from build123d import *

# Parameters (mm, degrees)
SKETCH1_R           = 13.75
SKETCH1_R_2         = 4.15
BOSS_EXTRUDE1_DEPTH = 2.5
SKETCH2_R           = 6.5
SKETCH2_R_2         = 4.15
BOSS_EXTRUDE2_DEPTH = 2.5
CUT_EXTRUDE1_DEPTH  = 21.077973005
FILLET1_R           = 0.5


with BuildPart() as part:
    # Sketch1 → Boss-Extrude1 (new body)
    with BuildSketch(Plane.XY):
        Circle(SKETCH1_R)
        Circle(SKETCH1_R_2, mode=Mode.SUBTRACT)
    extrude(amount=BOSS_EXTRUDE1_DEPTH)

    # Sketch2 → Boss-Extrude2 (add)
    with BuildSketch(Plane.XY.offset(2.5)):
        Circle(SKETCH2_R)
        Circle(SKETCH2_R_2, mode=Mode.SUBTRACT)
    extrude(amount=BOSS_EXTRUDE2_DEPTH)

    # Sketch5 → Cut-Extrude1 (cut, through all)
    with BuildSketch(Plane.XY):
        with BuildLine():
            Line((0, 12.75), (0, 7.5))
            ThreePointArc((0, 7.5), (5.303300859, 5.303300859), (7.5, 0))
            ThreePointArc((7.5, 0), (5.303300859, -5.303300859), (0, -7.5))
            Line((0, -7.5), (0, -12.75))
            ThreePointArc((0, -12.75), (9.01561146, -9.01561146), (12.75, 0))
            ThreePointArc((12.75, 0), (9.01561146, 9.01561146), (0, 12.75))
        make_face()
    extrude(amount=CUT_EXTRUDE1_DEPTH, mode=Mode.SUBTRACT)

    # Fillet1
    fillet1_edges = [part.edges().sort_by_distance(p)[0] for p in [
        (0, 7.5, 1.25),
        (0, -7.5, 1.25),
        (0, -12.75, 1.25),
        (0, 12.75, 1.25),
    ]]
    fillet(fillet1_edges, radius=FILLET1_R)


solid = part.part
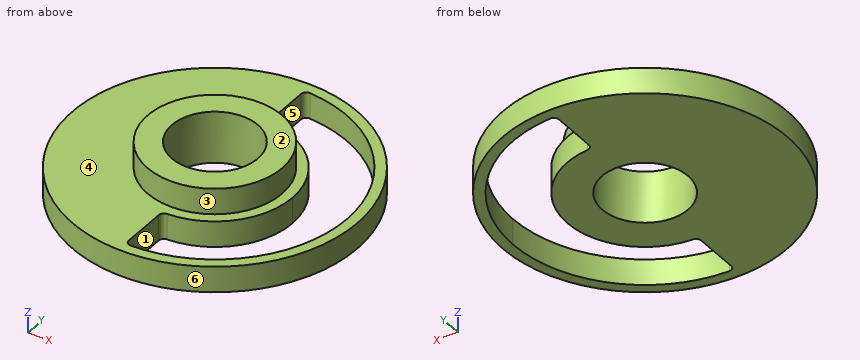
CAD build for the part. Positions are in the model's coordinates, mm. Face numbers are marked on the shaded views. A direction names the side the tool comes from. Coordinates: 2 decimals unless noted, no trailing zeros. Write each loop counter-clockwise with the first axis right and the second up, starting at its lowest first coordinate (ties: lowest second). Pieces come first, ordered by that corner, then holes. Notation, with made-up numbers: M 36,7 L 76,7 A19 cw 76,35 Z; hole C -14,57 d1. An arc over 180 degrees is marked long. Answer as a JSON object with one key per item and string values. Group by question number.
1) Wall check: line 1 (Y direction, x = 0, z = 4); line 2 (Y direction, x = 2.75, z = 1.1); line 3 (Z direction, x = -3.75, y = -12). Give the ranges that are in metal, low to high. Write a range as from..to.
2) Saw through at B-B (y = 3.75). Write the cut outline in (x, z).
3) Tool access for the marked faces 1, 2 and 3: list every direction of +Z, -Z, +X, -X, +Y, -Y with a clear straight run to the whole face (end or side of a thin tool).
4) Saw through at D-D (x = 3). Write the cut outline in (y, z), plus the area to 3 significant figures.
5) Saw through at C-C (x = 11). Write the cut outline in (y, z).
6) Mould opens along X. For the marked faces 4, 5 and 6 say: +X half, -X half, draft (parallel to the pull), parting line (faces both ways), or undercut.
7) Saw through at A-A (z = 1.5). Write the cut outline in (x, y), plus the area to 3 significant figures.
8) Pin check, flat tips, straight feed: pin 1 Ø2 at (x, z) = (-7, 4) entering from +Y; pin 2 Ø3 at (y, z) = (4, 2.5) entering from -X; pin 3 Ø2 at (x, z) = (-6, 3) entering from +Y; pin 4 Ø3 at (x, y) = (-4, -8.5) entering from -Z. Stop position of each tip, or through.
Values follow:
{
 "1": {"line 1": "y = -6.5..-4.15, 4.15..6.5", "line 2": "y = -13.47..-12.45, -6.98..-3.11, 3.11..6.98, 12.45..13.47", "line 3": "z = 0..2.5"},
 "2": {"outline": "M -13.23,0 L -1.78,0 L -1.78,5 L -5.31,5 L -5.31,2.5 L -13.23,2.5 Z; M 1.78,0 L 6.5,0 L 6.5,2.5 L 5.31,2.5 L 5.31,5 L 1.78,5 Z; M 12.19,0 L 13.23,0 L 13.23,2.5 L 12.19,2.5 Z"},
 "3": {"face 1": "+Z, -Z", "face 2": "+Z, +X, -X, +Y, -Y", "face 3": "+Z"},
 "4": {"outline": "M -13.42,0 L -12.39,0 L -12.39,2.5 L -13.42,2.5 Z; M -6.87,0 L -2.87,0 L -2.87,5 L -5.77,5 L -5.77,2.5 L -6.87,2.5 Z; M 2.87,0 L 6.87,0 L 6.87,2.5 L 5.77,2.5 L 5.77,5 L 2.87,5 Z; M 12.39,0 L 13.42,0 L 13.42,2.5 L 12.39,2.5 Z", "area": "39.7 mm2"},
 "5": {"outline": "M -8.25,0 L -6.45,0 L -6.45,2.5 L -8.25,2.5 Z; M 6.45,0 L 8.25,0 L 8.25,2.5 L 6.45,2.5 Z"},
 "6": {"face 4": "draft", "face 5": "undercut", "face 6": "parting line"},
 "7": {"outline": "C 0,0 d27.5; hole C 0,0 d8.3; hole M 0,-12.24 A0.5 ccw 0.52,-12.74 A12.75 ccw 0.52,12.74 A0.5 ccw 0,12.24 L 0,7.98 A0.5 ccw 0.47,7.49 A7.5 cw 0.47,-7.49 A0.5 ccw 0,-7.98 Z", "area": "373 mm2"},
 "8": {"pin 1": "stops at y = 2.5", "pin 2": "stops at x = -13.52", "pin 3": "stops at y = 12.76", "pin 4": "stops at z = 0"}
}
